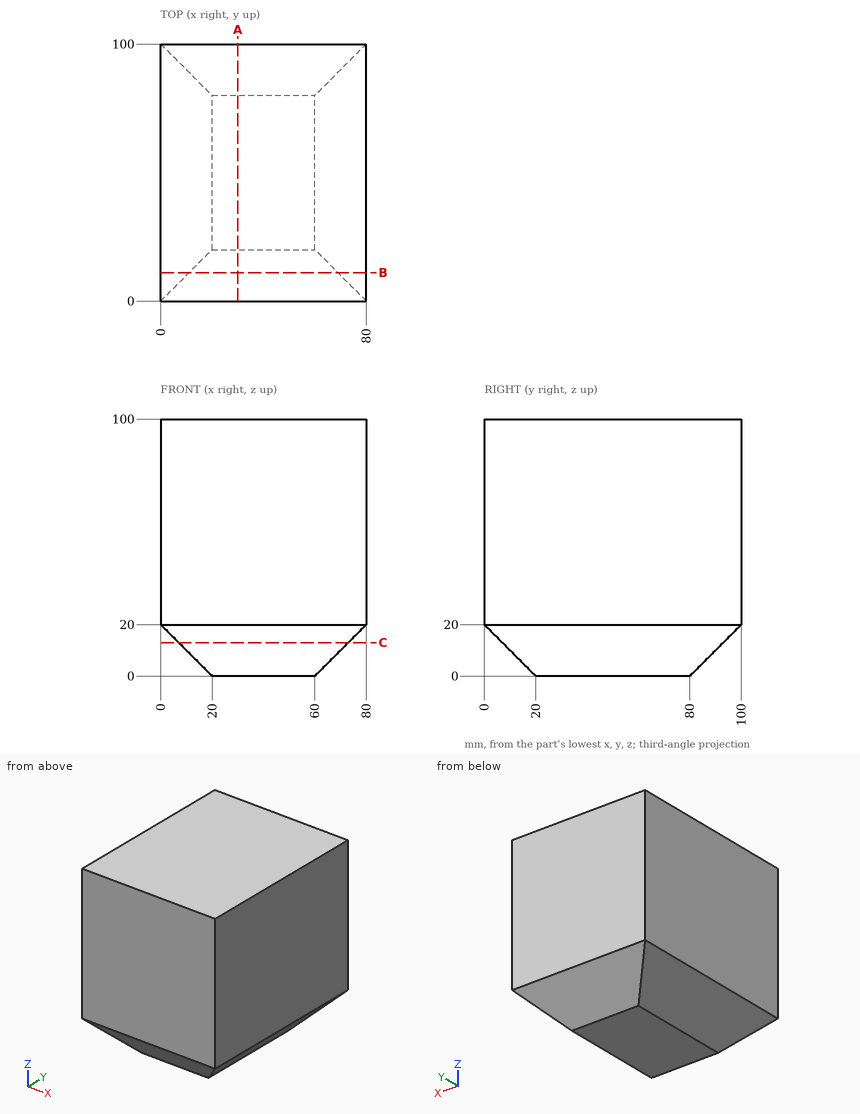
The figure shows three views and two pictorial views of one solid part (mm, origin at its lowest corner). Answer the questions. Round coordinates to 2 decimals unless told otherwise and drop trailing zeros. Loops run counter-clockwise (first coordinate to the right, second up) from the corner with the lowest first, then second, coordinate; pieces in that order, holes last. Notation, with made-up numbers: (82, 74) - (135, 74) arc R14 cw to (135, 97) - close; hole circle Ø5 at (-11, -30). An arc over 180 degrees is marked (long way). Use one line per item in the form item = value. Start each with the question number.
(1) Consider line 1 (Z direction, x = 65.5, y = 63); line 2 (Z direction, x = 15.5, y = 8); line 3 (X direction, y = 15.5, z = 6). Determine where each line is inside the solid, lowest interval first.
(2) A flat-ended cylindrical pin translates along its axis: P1, Ø4, axis at x = 22, z = 43.5, coming from the -Y side. Find the tip coordinate at first contact, or state that the pin passes through.
(3) Find section C-C on z = 13. Determine the outline of the cut face in (x, y).
(4) Find section B-B on y = 11. Determine the outline of the cut face in (x, z), and give its area (3 significant figures).
(5) Find section A-A on x = 30. Determine the outline of the cut face in (y, z), and give its area (3 significant figures).
Answer list:
q1.line_1 = 5.5 to 100
q1.line_2 = 12 to 100
q1.line_3 = 14 to 66
q2.P1 = 0
q3.outline = (7, 7) - (73, 7) - (73, 93) - (7, 93) - close
q4.outline = (0, 20) - (11, 9) - (69, 9) - (80, 20) - (80, 100) - (0, 100) - close
q4.area = 7,160 mm^2
q5.outline = (0, 20) - (20, 0) - (80, 0) - (100, 20) - (100, 100) - (0, 100) - close
q5.area = 9,600 mm^2
